from build123d import *

# Parameters (mm, degrees)
SKETCH1_W               = 20.894747592
SKETCH1_H               = 135.476524453
BOSS_EXTRUDE1_DEPTH     = 3.175
SKETCH2_R               = 2.912030795
CUT_EXTRUDE2_DEPTH      = 1
CUT_EXTRUDE2_DEPTH_BACK = 4.175
SKETCH2_4_R             = 3.450024598
BOSS_EXTRUDE2_DEPTH     = 9.652
BOSS_EXTRUDE3_DEPTH     = 1.27


with BuildPart() as part:
    # Sketch1 → Boss-Extrude1 (new body)
    with BuildSketch(Plane.XY):
        with Locations((-10.447373796, 67.738262226)):
            Rectangle(SKETCH1_W, SKETCH1_H)
    extrude(amount=BOSS_EXTRUDE1_DEPTH)

    # Sketch2 → Cut-Extrude2 (cut, two sides)
    with BuildSketch(Plane(origin=(0, 0, 0), x_dir=(-1, 0, 0), z_dir=(0, 0, -1))) as cut_extrude2_sk:
        with Locations((10.447373796, 6.305347679)):
            Circle(SKETCH2_R)
    extrude(amount=CUT_EXTRUDE2_DEPTH, mode=Mode.SUBTRACT)
    extrude(cut_extrude2_sk.sketch, amount=-CUT_EXTRUDE2_DEPTH_BACK, mode=Mode.SUBTRACT)

    # Sketch2<4> → Boss-Extrude2 (add)
    with BuildSketch(Plane(origin=(0, 0, 0), x_dir=(-1, 0, 0), z_dir=(0, 0, -1))):
        with Locations((15.198897526, 22.445779357)):
            Circle(SKETCH2_4_R)
    extrude(amount=BOSS_EXTRUDE2_DEPTH)

    # Sketch3 → Boss-Extrude3 (add)
    with BuildSketch(Plane(origin=(0, 0, -9.652), x_dir=(-1, 0, 0), z_dir=(0, 0, -1))):
        Polygon((10.964889393, 25.99164554), (10.011083267, 20.551953845), (14.2450914, 17.006087662), (19.432905659, 18.899913174), (20.386711785, 24.339604868), (16.152703653, 27.885471051), align=None)
    extrude(amount=BOSS_EXTRUDE3_DEPTH)


solid = part.part
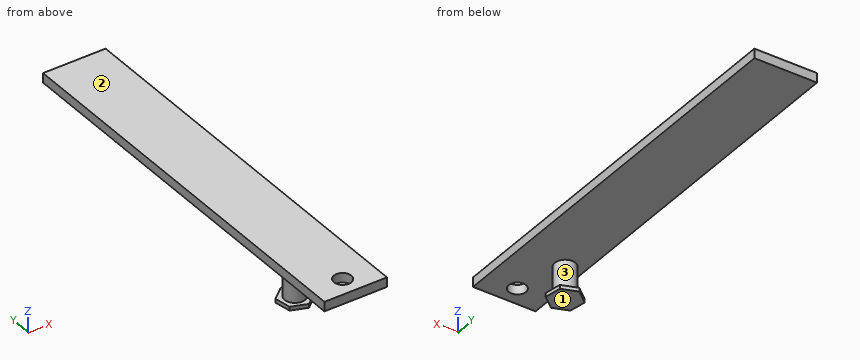
Work out the finished part from the listing and answer in its coordinate system (mm). Face numbers are marked on the shaded views. Coordinates: 2 decimals unless noted, no trailing zeros. Loops run counter-clockwise (first coordinate to the right, second up) from the corner with the lowest first, then second, coordinate; pieces in that order, holes last. Notation, with made-up numbers: (20, 52.25) -> (37, 52.25) arc R19 cw to (37, 80.25) -> close; hole circle Ø11 at (89, 84.25). An arc over 180 degrees is marked (long way). Answer as CSV lines item,"result".
1) The part is cut by section B-B (y = 87). Give the vertices of the cut face in (x, z) (3 decimals).
A:
outline,"(-20.895, 0) -> (0, 0) -> (0, 3.175) -> (-20.895, 3.175) -> close"
2) Straight lines are drawn through the part: probe 1 along Z at (x, y) = (-12.75, 49) (3 decimals); probe 2 along Y at (x, z) = (-8.75, 0.25); probe 3 along Y at (x, z) = (-16.5, -5.25). For each, find the intervals that lie inside material, in ascending order.
A:
probe 1,"z = 0 to 3.175"
probe 2,"y = 0 to 3.94, 8.67 to 135.48"
probe 3,"y = 19.25 to 25.64"
3) The part is cut by section A-A (x = -6). Give the vertices of the cut face in (y, z) (3 decimals), and give its area (3 significant figures).
A:
outline,"(0, 0) -> (135.477, 0) -> (135.477, 3.175) -> (0, 3.175) -> close"
area,"430 mm²"
4) For a pull along Z with two mould halves and no side action, classify the marked faces 1, 2 and 3 as released by +Z, released by -Z, zero draft, split by the parting line, or undercut.
A:
face 1,"released by -Z"
face 2,"released by +Z"
face 3,"undercut"
5) The part is cut by section C-C (z = -6.75). Give the vertices of the cut face in (x, y), and give its area (3 significant figures).
A:
outline,"circle Ø6.9 at (-15.2, 22.45)"
area,"37.4 mm²"
6) Flat-ended cylindrical pins translate along their axes: pin 1 (10 mm diameter, centred on x = -9, y = 65, fed in from -Z); pin 2 (3.5 mm diameter, centred on x = -10.45, y = 6.31, fed in from -Z). Find the tip coordinate at first contact, or state that the pin passes through.
A:
pin 1,"stops at z = 0"
pin 2,"passes through"
